```python
from build123d import *

# Parameters (mm, degrees)
F0_W     = 101.6
F0_H     = 101.6
F1_DEPTH = 101.6
F2_W     = 10.4571996808
F2_H     = 7.7591115123
F2_W_2   = 24.1928109899
F2_H_2   = 19.4694609827
F2_W_3   = 11.7103494704
F2_H_3   = 16.3430143148
F2_W_4   = 20.3322558664
F2_H_4   = 24.7075520456
F3_DEPTH = 25.4
F2_W_5   = 51.507767962
F2_H_5   = 7.5924228877
F4_DEPTH = 25.4
F5_W     = 28.8430942774
F5_H     = 24.771893397
F6_DEPTH = 25.4
F5_W_2   = 87.2339873195
F5_H_2   = 1.1734974742
F7_DEPTH = 25.4


with BuildPart() as f1:
    # F0 (on Front) → F1 (new body)
    with BuildSketch(Plane.XZ):
        with Locations((0.8686259389, 4.0604042715)):
            Rectangle(F0_W, F0_H)
    extrude(amount=-F1_DEPTH)

    # F2 (on face) → F3 (cut)
    with BuildSketch(Plane.XZ):
        with Locations((-44.7027742207, 50.9808485153)):
            Rectangle(F2_W, F2_H)
        with Locations((0.8042831905, 45.1256737802)):
            Rectangle(F2_W_2, F2_H_2)
        with Locations((-30.9166107327, 29.6644521877)):
            Rectangle(F2_W_3, F2_H_3)
        with Locations((-16.0534728784, -19.1715676337)):
            Rectangle(F2_W_4, F2_H_4)
        Polygon((19.9783723801, -14.9249564856), (19.9783723801, -46.7395957285), (51.6686259389, -46.7395957285), (51.6686259389, -28.5655856133), (37.6082397997, -28.5655856133), (44.6859262884, -14.9249564856), align=None)
    extrude(amount=-F3_DEPTH, mode=Mode.SUBTRACT)

    # F2 (on face) → F4 (join)
    with BuildSketch(Plane.XZ):
        Polygon((-24.4180094451, 11.84155792), (-34.8415076733, 7.9810023308), (-41.2757657468, 2.447540639), (-32.9112298787, -6.4317355864), (4.7935228795, 0.5172632518), align=None)
        with Locations((25.9147419579, 22.3293984309)):
            Rectangle(F2_W_5, F2_H_5)
    extrude(amount=F4_DEPTH)

    # F5 (on face) → F6 (join)
    with BuildSketch(Plane.XY.offset(54.8604042715)):
        with Locations((37.2470788002, 43.1616036221)):
            Rectangle(F5_W, F5_H)
        Polygon((-23.9836964756, 77.4240270257), (-49.9313740611, 55.0649799407), (-49.9313740611, 45.5744490027), (-22.5359871984, 42.6790341735), (-10.4717537761, 72.9200467467), (-37.4956354499, 52.1695651114), align=None)
    extrude(amount=F6_DEPTH)

    # F5 (on face) → F7 (cut)
    with BuildSketch(Plane.XY.offset(54.8604042715)):
        with Locations((-6.3143804014, 101.0132512629)):
            Rectangle(F5_W_2, F5_H_2)
        Polygon((17.3564106226, 57.638682425), (21.3778242469, 76.4588862658), (8.8310204446, 68.7377750874), (6.418173667, 57.638682425), align=None)
    extrude(amount=-F7_DEPTH, mode=Mode.SUBTRACT)


solid = f1.part
```
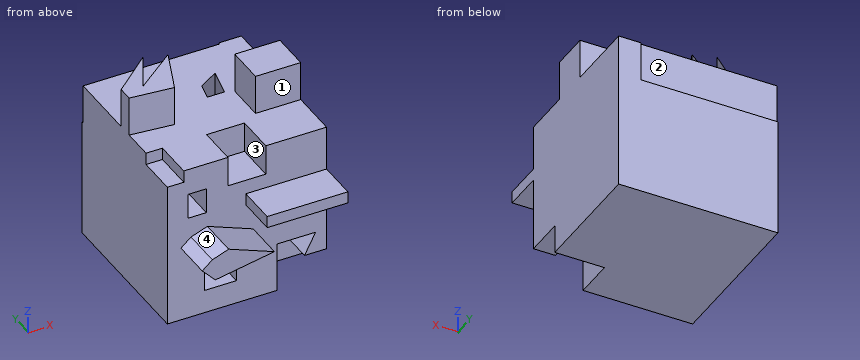
Geometry check sheet. Reference: the model listing, model coordinates, mm. Face numbers are marked on the shaded views. A direction names the side the tool comes from. Round coordinates to 2 decimals unless told otherwise and drop trailing zeros. Loops run counter-clockwise (first coordinate to the right, second up) from the corner with the lowest first, then second, coordinate; pieces in that order, holes last. Notation, with made-up numbers: (64.5, 76.5) - (95.5, 76.5) arc R32 cw to (95.5, 106.5) - close; hole circle Ø11 at (39.5, 71). An arc over 180 degrees is marked (long way). Write each question's results on one line, items separated by ' | '. Start each with the question number.
Q1. Cross-section at C-C on y = 10.5. Enter the section's corners in (x, z).
Q2. Gauge pin test, flat ends, axial feed: P1, Ø16, axis at x = 36.5, z = -25.5, coming from the -Y side; P2, Ø5, axis at x = -24, y = -6.5, coming from the -Z side; P3, Ø19.5, axis at x = 2.5, y = 12.5, coming from the +Z side. Record the tip position at first contact, or that the pin passes through.
Q3. Cross-section at A-A on z = 49.5. Enter the section's corners in (x, y).
Q4. Cross-section at D-D on z = -8.5. Enter the section's corners in (x, y), and give its area (3 significant figures).
Q5. Thickness scan on line 1 (X direction, y = 1, z = -19); line 2 (X direction, y = 8.5, z = 41); line 3 (Y direction, x = -8, z = 41). Record the ranges inside material, lowest first. Write a range as [from, to].
Q6. Cross-section at B-B on y = -14.5. Enter the section's corners in (x, z).
Q7. Access from +Z, -Z, +X, -X, +Y, -Y to the whole of each face (thin tool, end or side, straight path). Record for the marked faces 1, 2, 3 and 4.
Answers below:
1) outline: (-49.93, -46.74) - (19.98, -46.74) - (19.98, -14.92) - (44.69, -14.92) - (37.61, -28.57) - (51.67, -28.57) - (51.67, 54.86) - (12.9, 54.86) - (12.9, 35.39) - (-11.29, 35.39) - (-11.29, 54.86) - (-39.47, 54.86) - (-39.47, 47.1) - (-49.93, 47.1) - close; hole (-36.77, 21.49) - (-25.06, 21.49) - (-25.06, 37.84) - (-36.77, 37.84) - close; hole (-26.22, -31.53) - (-5.89, -31.53) - (-5.89, -6.82) - (-26.22, -6.82) - close
2) P1: stops at y = 0 | P2: stops at z = -5.25 | P3: stops at z = 35.39
3) outline: (-49.93, 25.4) - (-39.47, 25.4) - (-39.47, 0) - (-11.29, 0) - (-11.29, 25.4) - (12.9, 25.4) - (12.9, 0) - (51.67, 0) - (51.67, 101.6) - (37.3, 101.6) - (37.3, 100.43) - (-49.93, 100.43) - close; hole (6.42, 57.64) - (17.36, 57.64) - (21.38, 76.46) - (8.83, 68.74) - close
4) outline: (-49.93, 0) - (-26.22, 0) - (-26.22, 25.4) - (-5.89, 25.4) - (-5.89, 0) - (51.67, 0) - (51.67, 101.6) - (-49.93, 101.6) - close | area: 9,810 mm²
5) line 1: x = [-49.93, -26.22], [-5.89, 19.98], [42.57, 51.67] | line 2: x = [-49.93, -11.29], [12.9, 51.67] | line 3: y = [25.4, 100.43]
6) outline: (-41.28, 2.45) - (-32.91, -6.43) - (4.79, 0.52) - (-24.42, 11.84) - (-34.84, 7.98) - close; (0.16, 18.53) - (51.67, 18.53) - (51.67, 26.13) - (0.16, 26.13) - close
7) face 1: +Z, +X, -X, -Y | face 2: +Z, -X, +Y | face 3: +Z, -Y | face 4: +Z, -X, -Y
